Check sheet for the modelled part. Datum: model origin and axes. Units: mm. A direction names the side the tool comes from. Coordinates: 2 decimals unless noted, no trailing zeros. Loops run counter-clockwise (first coordinate to the right, second up) from the corner with the lowest first, then second, coordinate; pieces in that order, holes last. Notation, with made-up numbers: M 32.25,87 L 47.25,87 A23 ccw 47.25,102 Z; hole C -38,35.5 d6. An arc over 180 degrees is marked long. Return JSON: item names as keys, results as strings.
from build123d import *

# Parameters (mm, degrees)
SKETCH1_W           = 28.5
SKETCH1_H           = 22
SKETCH1_R           = 1.5
BOSS_EXTRUDE1_DEPTH = 1.5
SKETCH1_3_W         = 1.5
SKETCH1_3_H         = 22
BOSS_EXTRUDE2_DEPTH = 15


with BuildPart() as part:
    # Sketch1 → Boss-Extrude1 (new body)
    with BuildSketch(Plane(origin=(0, 0, 0), x_dir=(1, 0, 0), z_dir=(0, 1, 0))):
        with Locations((0.75, 0)):
            Rectangle(SKETCH1_W, SKETCH1_H)
        with Locations(Location((1.435, 1, 0), (0, 0, 270))):
            Circle(SKETCH1_R, mode=Mode.SUBTRACT)
    extrude(amount=-BOSS_EXTRUDE1_DEPTH)

    # Sketch1_3 → Boss-Extrude2 (add)
    with BuildSketch(Plane(origin=(0, 0, 0), x_dir=(1, 0, 0), z_dir=(0, 1, 0))):
        with Locations((-14.25, 0)):
            Rectangle(SKETCH1_3_W, SKETCH1_3_H)
    extrude(amount=-BOSS_EXTRUDE2_DEPTH)


solid = part.part
1) Section check B-B on y = -10. Record the cut outline in (x, z), then the cut area to 3 significant figures.
Answers:
{"outline": "M -15,-11 L -13.5,-11 L -13.5,11 L -15,11 Z", "area": "33.0 mm²"}
2) Section check C-C on x = -8. Record the cut outline in (y, z), then the cut area to 3 significant figures.
Answers:
{"outline": "M -1.5,-11 L 0,-11 L 0,11 L -1.5,11 Z", "area": "33.0 mm²"}
3) Set-up check for faces 4 (the face through (0, 0, 0)), 5 (the face through (1, -1.5, -3)): record each of +Z, -Z, +X, -X, +Y, -Y from which the full face is reachable in a straight line by a thin tool's end or side.
Answers:
{"face 4": "+Z, -Z, +X, -X, +Y", "face 5": "+Z, -Z, +X, -Y"}
4) Draft check along X on faces 1 (the face through (15, -1, 0)), 2 (the face through (-14, -15, 0)), 3 (the face through (-0.03, -0.74, -1.33)). Enter one of: +X half, -X half, draft (parallel to the pull), parting line (faces both ways), or undercut.
Answers:
{"face 1": "+X half", "face 2": "draft", "face 3": "undercut"}
5) Scan lines: line 1 along X through (y, z) = (-0.4, -1) (3 decimals); line 2 along X through (y, z) = (-7.25, 0); line 3 along Y through (x, z) = (-8, -1). Record each from-to range of solid material in increasing order. Write a range as [from, to].
Answers:
{"line 1": "[-15, -0.065], [2.935, 15]", "line 2": "[-15, -13.5]", "line 3": "[-1.5, 0]"}
6) Go/stop test with flat-tipped pins: pin 1 Ø4 at (y, z) = (-5, -4.5) entering from +X; pin 2 Ø1 at (x, z) = (7, 0) entering from -Y; pin 3 Ø2.5 at (x, z) = (1.435, -1) entering from +Y. Record where each tip stops, or that it passes through.
Answers:
{"pin 1": "x = -13.5", "pin 2": "y = -1.5", "pin 3": "through"}
7) Section check A-A on z = -1. Record the cut outline in (x, y) (3 decimals).
Answers:
{"outline": "M -15,-15 L -13.5,-15 L -13.5,-1.5 L -0.065,-1.5 L -0.065,0 L -15,0 Z; M 2.935,-1.5 L 15,-1.5 L 15,0 L 2.935,0 Z"}
